Part model, mm, in its own coordinate system. Face numbers are marked on the shaded views. A direction names the side the tool comes from. Give positions to 0.01 mm unless a question says otherwise; leave off trailing zeros. Order: outer loops, then holes, each group sorted by start corner. A loop starts at its lowest first (then second) coordinate and runs counter-clockwise, first axis right, second up. Notation, with made-up numbers: M 47,7.5 L 68,7.5 A20 ccw 68,21.5 Z; hole C -5,29 d3. An arc over 180 degrees is marked long. Answer as a JSON object with one key per item and string values.
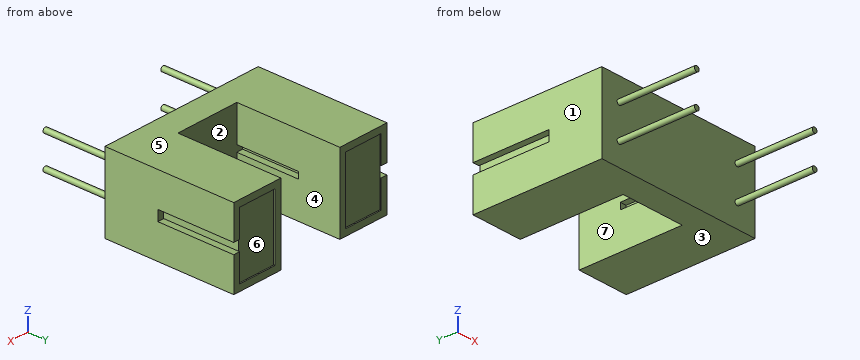
from build123d import *

# Parameters (mm, degrees)
ESBO_O2_W                = 13
ESBO_O2_H                = 6
RESSALTO_EXTRUS_O1_DEPTH = 10
ESBO_O3_W                = 5
ESBO_O3_H                = 6
CORTE_EXTRUS_O1_DEPTH    = 8
ESBO_O4_W                = 3
ESBO_O4_H                = 5
CORTE_EXTRUS_O2_DEPTH    = 0.1
ESBO_O5_W                = 1
ESBO_O5_H                = 0.8
CORTE_EXTRUS_O3_DEPTH    = 5.9
ESBO_O6_W                = 1
ESBO_O6_H                = 0.5
CORTE_EXTRUS_O4_DEPTH    = 4.8
ESBO_O7_R                = 0.2
RESSALTO_EXTRUS_O2_DEPTH = 6


with BuildPart() as part:
    # Esboço2 → Ressalto-extrusão1 (new body)
    with BuildSketch(Plane(origin=(0, 0, 0), x_dir=(1, 0, 0), z_dir=(0, 1, 0))):
        Rectangle(ESBO_O2_W, ESBO_O2_H)
    extrude(amount=RESSALTO_EXTRUS_O1_DEPTH)

    # Esboço3 → Corte-extrusão1 (cut)
    with BuildSketch(Plane(origin=(0, 10, 0), x_dir=(1, 0, 0), z_dir=(0, 1, 0))):
        Rectangle(ESBO_O3_W, ESBO_O3_H)
    extrude(amount=-CORTE_EXTRUS_O1_DEPTH, mode=Mode.SUBTRACT)

    # Esboço4 → Corte-extrusão2 (cut)
    with BuildSketch(Plane(origin=(0, 10, 0), x_dir=(1, 0, 0), z_dir=(0, 1, 0))):
        with Locations((-4.5, 0)):
            Rectangle(ESBO_O4_W, ESBO_O4_H)
    corte_extrus_o2 = extrude(amount=-CORTE_EXTRUS_O2_DEPTH, mode=Mode.SUBTRACT)

    # Espelhar1: Corte-extrusão2 across plane
    add(corte_extrus_o2.mirror(Plane(origin=(0, 0, 0), x_dir=(0, 0, 1), z_dir=(1, 0, 0))), mode=Mode.SUBTRACT)

    # Esboço5 → Corte-extrusão3 (cut)
    with BuildSketch(Plane(origin=(0, 10, 0), x_dir=(1, 0, 0), z_dir=(0, 1, 0))):
        with Locations((-6.5, 0)):
            Rectangle(ESBO_O5_W, ESBO_O5_H)
    corte_extrus_o3 = extrude(amount=-CORTE_EXTRUS_O3_DEPTH, mode=Mode.SUBTRACT)

    # Espelhar2: Corte-extrusão3 across plane
    add(corte_extrus_o3.mirror(Plane(origin=(0, 0, 0), x_dir=(0, 0, 1), z_dir=(1, 0, 0))), mode=Mode.SUBTRACT)

    # Esboço6 → Corte-extrusão4 (cut)
    with BuildSketch(Plane(origin=(0, 6.8, 0), x_dir=(1, 0, 0), z_dir=(0, 1, 0))):
        with Locations((-2.5, 0)):
            Rectangle(ESBO_O6_W, ESBO_O6_H)
    corte_extrus_o4 = extrude(amount=-CORTE_EXTRUS_O4_DEPTH, mode=Mode.SUBTRACT)

    # Espelhar3: Corte-extrusão4 across plane
    add(corte_extrus_o4.mirror(Plane(origin=(0, 0, 0), x_dir=(0, 0, 1), z_dir=(1, 0, 0))), mode=Mode.SUBTRACT)

    # Esboço7 → Ressalto-extrusão2 (add)
    with BuildSketch(Plane.XZ):
        with Locations((-5, 1.27)):
            Circle(ESBO_O7_R)
        with Locations((5, 1.27)):
            Circle(ESBO_O7_R)
        with Locations((5, -1.27)):
            Circle(ESBO_O7_R)
        with Locations((-5, -1.27)):
            Circle(ESBO_O7_R)
    extrude(amount=RESSALTO_EXTRUS_O2_DEPTH)


solid = part.part
1. Two-plate mould, pull along X, no slides. Class the marked faces 1, 2, 3 and 4: +X half, -X half, draft (parallel to the pull), parting line (faces both ways), or undercut.
Worked answers:
{"face 1": "-X half", "face 2": "undercut", "face 3": "draft", "face 4": "undercut"}
2. Cut at B-B on y = 5.25. Give the cut face in (x, z).
Worked answers:
{"outline": "M -6.5,-3 L -2.5,-3 L -2.5,-0.25 L -3,-0.25 L -3,0.25 L -2.5,0.25 L -2.5,3 L -6.5,3 L -6.5,0.4 L -6,0.4 L -6,-0.4 L -6.5,-0.4 Z; M 2.5,-3 L 6.5,-3 L 6.5,-0.4 L 6,-0.4 L 6,0.4 L 6.5,0.4 L 6.5,3 L 2.5,3 L 2.5,0.25 L 3,0.25 L 3,-0.25 L 2.5,-0.25 Z"}
3. Which spindle directions (+Z, -Z, +X, -X, +Y, -Y) get a long thin tool onto all of the face, cutting with end or side? Do the marked faces 5, 6 and 7. Say none if no direction does.
Worked answers:
{"face 5": "+Z, +X, -X, +Y, -Y", "face 6": "+Y", "face 7": "+Z, -Z, +Y"}
4. Probe line 1 along X through (y, z) = (4, -0.95); line 2 along X through (y, z) = (3, 0.2); line 3 along Z through (x, y) = (5, -0.75). List the from-to ranges inside material, lowest first.
Worked answers:
{"line 1": "x = -6.5 to -2.5, 2.5 to 6.5", "line 2": "x = -6.5 to -3, 3 to 6.5", "line 3": "z = -1.47 to -1.07, 1.07 to 1.47"}
5. Cut at A-A on y = 9. Give the cut face in (x, z), plus the area to 3 significant figures.
Worked answers:
{"outline": "M -6.5,-3 L -2.5,-3 L -2.5,3 L -6.5,3 L -6.5,0.4 L -6,0.4 L -6,-0.4 L -6.5,-0.4 Z; M 2.5,-3 L 6.5,-3 L 6.5,-0.4 L 6,-0.4 L 6,0.4 L 6.5,0.4 L 6.5,3 L 2.5,3 Z", "area": "47.2 mm^2"}
6. Cut at C-C on x = -5. Give the cut face in (y, z).
Worked answers:
{"outline": "M -6,-1.47 L 0,-1.47 L 0,-3 L 10,-3 L 10,-2.5 L 9.9,-2.5 L 9.9,2.5 L 10,2.5 L 10,3 L 0,3 L 0,1.47 L -6,1.47 L -6,1.07 L 0,1.07 L 0,-1.07 L -6,-1.07 Z"}
7. Pin check, flat tips, straight feed: P1, Ø0.6, axis at y = 4.5, z = 0, coming from the -X side; P2, Ø1, axis at x = -4.5, y = -2.5, coming from the +Z side; P3, Ø0.6, axis at x = -6.5, z = 0, coming from the +Y side; P4, Ø2.5, axis at x = 5, z = 0, coming from the +Y side. Stop position of each tip, or through.
Worked answers:
{"P1": "stops at x = -6", "P2": "stops at z = 1.47", "P3": "stops at y = 4.1", "P4": "stops at y = 10"}
8. Cut at D-D on z = 1.27. Give the cut face in (x, y), plus the area to 3 significant figures.
Worked answers:
{"outline": "M -6.5,0 L -5.2,0 L -5.2,-6 L -4.8,-6 L -4.8,0 L 4.8,0 L 4.8,-6 L 5.2,-6 L 5.2,0 L 6.5,0 L 6.5,10 L 6,10 L 6,9.9 L 3,9.9 L 3,10 L 2.5,10 L 2.5,2 L -2.5,2 L -2.5,10 L -3,10 L -3,9.9 L -6,9.9 L -6,10 L -6.5,10 Z", "area": "94.2 mm^2"}
